```python
from build123d import *

# Parameters (mm, degrees)
SKETCH_1_R          = 1.5
SKETCH_1_W          = 10
SKETCH_1_H          = 16
EXTRUDE_1_DEPTH     = 1.5
SKETCH_2_R          = 1.5
CUT_EXTRUDE_1_DEPTH = 10


with BuildPart() as part:
    # 草图1 → 凸台-拉伸1 (new body)
    # profile 1 of 2: a face of its own
    with BuildSketch(Plane.XY):
        Polygon((-13.65, 28.439884515), (-13.65, 14.6), (-13.65, -14.6), (13.65, -14.6), (13.65, 14.6), (13.65, 28.439884515), align=None)
        with Locations((0, -12.560115485)):
            Circle(SKETCH_1_R, mode=Mode.SUBTRACT)
        with Locations((0, -0.560115485)):
            Rectangle(SKETCH_1_W, SKETCH_1_H, mode=Mode.SUBTRACT)
    # profile 2 of 2: a face of its own
    with BuildSketch(Plane.XY):
        Polygon((-13.65, 28.439884515), (-13.65, 14.6), (-13.65, -14.6), (13.65, -14.6), (13.65, 14.6), (13.65, 28.439884515), align=None)
        with Locations((0, -12.560115485)):
            Circle(SKETCH_1_R, mode=Mode.SUBTRACT)
        with Locations((0, -0.560115485)):
            Rectangle(SKETCH_1_W, SKETCH_1_H, mode=Mode.SUBTRACT)
    extrude(amount=EXTRUDE_1_DEPTH)

    # 草图2 → 切除-拉伸1 (cut)
    with BuildSketch(Plane(origin=(0, 0, 0), x_dir=(-1, 0, 0), z_dir=(0, 0, -1))):
        with Locations((0, 26.068537202)):
            Circle(SKETCH_2_R)
    extrude(amount=-CUT_EXTRUDE_1_DEPTH, mode=Mode.SUBTRACT)


solid = part.part
```
Input: part model. Units: mm. Frame: model coordinates. A direction names the side the tool comes from. Give positions to 0.01 mm unless a question says otherwise; leave off trailing zeros. Loops run counter-clockwise (first coordinate to the right, second up) from the corner with the lowest first, then second, coordinate; pieces in that order, holes last. Notation, with made-up numbers: (58.5, 81.25) -> (101.5, 81.25) arc R25 cw to (101.5, 96.25) -> close; hole circle Ø6 at (81, -2). An arc over 180 degrees is marked (long way). Use a Markdown table: item, result.
Q1. Pull-direction query (Y, two-part tool) for faces 1 (the flat face through (13.65, 7, 1)), 2 (the flat face through (0, 7.44, 1)), 3 (the flat face through (0, 28.44, 1)), 4 (the flat face through (0, -14.6, 1)); classes: pulls with the +Y half, pulls with the -Y half, needs draft (parallel to the pull), parting line crosses it, or undercut.
Entries:
| item | result |
|---|---|
| face 1 | needs draft |
| face 2 | undercut |
| face 3 | pulls with the +Y half |
| face 4 | pulls with the -Y half |
Q2. Section query A-A, the plane x = 4.25. Return the cut outline in (y, z).
Entries:
| item | result |
|---|---|
| outline | (-14.6, 0) -> (-8.56, 0) -> (-8.56, 1.5) -> (-14.6, 1.5) -> close; (7.44, 0) -> (28.44, 0) -> (28.44, 1.5) -> (7.44, 1.5) -> close |
Q3. Section query B-B, the plane y = 4.5. Return the cut outline in (x, z).
Entries:
| item | result |
|---|---|
| outline | (-13.65, 0) -> (-5, 0) -> (-5, 1.5) -> (-13.65, 1.5) -> close; (5, 0) -> (13.65, 0) -> (13.65, 1.5) -> (5, 1.5) -> close |
Q4. Access query for faces 5 (the flat face through (-13.65, 7, 1)), 6 (the flat face through (0, -8.56, 1)). Directions: +Z, -Z, +X, -X, +Y, -Y. A direction counts if a zero-diameter tool reaches every point of the face in a straight line with its end or side. Return the directions, or none.
Entries:
| item | result |
|---|---|
| face 5 | +Z, -Z, -X, +Y, -Y |
| face 6 | +Z, -Z |
Q5. First-contact query: P1, Ø1.8, axis at x = 0, y = -12.56, coming from the -Z side. Flat tip, straight axial feed; report the tip coordinate or a pass-through.
Entries:
| item | result |
|---|---|
| P1 | passes through |
Q6. Section query D-D, the plane z = 0.5. Return the cut outline in (x, y).
Entries:
| item | result |
|---|---|
| outline | (-13.65, -14.6) -> (13.65, -14.6) -> (13.65, 28.44) -> (-13.65, 28.44) -> close; hole (-5, -8.56) -> (5, -8.56) -> (5, 7.44) -> (-5, 7.44) -> close; hole circle Ø3 at (0, -12.56); hole circle Ø3 at (0, 26.07) |
Q7. Section query C-C, the plane x = 0. Return the cut outline in (y, z).
Entries:
| item | result |
|---|---|
| outline | (-14.6, 0) -> (-14.06, 0) -> (-14.06, 1.5) -> (-14.6, 1.5) -> close; (-11.06, 0) -> (-8.56, 0) -> (-8.56, 1.5) -> (-11.06, 1.5) -> close; (7.44, 0) -> (24.57, 0) -> (24.57, 1.5) -> (7.44, 1.5) -> close; (27.57, 0) -> (28.44, 0) -> (28.44, 1.5) -> (27.57, 1.5) -> close |
Q8. Ray query, probe 1 along Y at (x, z) = (0, 0.7); probe 2 along X at (y, z) = (26, 0.85); probe 3 along X at (y, z) = (0.5, 1.2). Return the intervals inside material, ascending. Write a range as from..to.
Entries:
| item | result |
|---|---|
| probe 1 | y = -14.6..-14.06, -11.06..-8.56, 7.44..24.57, 27.57..28.44 |
| probe 2 | x = -13.65..-1.5, 1.5..13.65 |
| probe 3 | x = -13.65..-5, 5..13.65 |
